```python
from build123d import *

# Parameters (mm, degrees)
SKETCH006_R     = 2.5
PAD002_DEPTH    = 9
SKETCH007_R     = 5.5
POCKET001_DEPTH = 1.85
SKETCH008_R     = 5.25
POCKET002_DEPTH = 67.1275389628
CHAMFER001_SIZE = 2.3


with BuildPart() as part:
    # Sketch006 → Pad002 (new body, symmetric)
    with BuildSketch(Plane.XY):
        with BuildLine():
            Line((20, -1.5), (20, 1.5))
            Line((20, 1.5), (7.1239047452, 1.5))
            ThreePointArc((3.9577107596, 3.0555728668), (5.3600599952, 1.9098946593), (7.1239047452, 1.5))
            ThreePointArc((3.9577107595, 3.0555728668), (-5, -2.4792e-06), (3.9577137897, -3.055568942))
            ThreePointArc((7.1239047446, -1.5), (5.3600622201, -1.9098935662), (3.9577137897, -3.055568942))
            Line((7.1239047446, -1.5), (20, -1.5))
        make_face()
        Circle(SKETCH006_R, mode=Mode.SUBTRACT)
    extrude(amount=PAD002_DEPTH, both=True)

    # Sketch007 → Pocket001 (cut, symmetric)
    with BuildSketch(Plane.XY):
        Circle(SKETCH007_R)
    extrude(amount=POCKET001_DEPTH, both=True, mode=Mode.SUBTRACT)

    # Sketch008 → Pocket002 (cut, through all)
    with BuildSketch(Plane.XY.offset(6.65)):
        Circle(SKETCH008_R)
    pocket002 = extrude(amount=POCKET002_DEPTH, mode=Mode.SUBTRACT)

    # Mirrored001: Pocket002 across XY
    add(pocket002.mirror(Plane.XY), mode=Mode.SUBTRACT)

    # Chamfer001
    chamfer001_edges = [part.edges().sort_by_distance(p)[0] for p in [
        (-2.5, 0, -6.65),
        (-2.5, 0, -1.85),
        (-2.5, 0, 6.65),
        (-2.5, 0, 1.85),
    ]]
    chamfer(chamfer001_edges, length=CHAMFER001_SIZE)


solid = part.part
```
Design review of the part built by this model. Coordinates are the model's own, in mm. A direction names the side the tool comes from. Give positions to 0.01 mm unless a question says otherwise; leave off trailing zeros. Write each loop counter-clockwise with the first axis right and the second up, starting at its lowest first coordinate (ties: lowest second). Pieces come first, ordered by that corner, then holes. Notation, with made-up numbers: (54.25, 42.5) - (64.25, 42.5) arc R24 ccw to (64.25, 52.5) - close; hole circle Ø4 at (83.5, 42.5). An arc over 180 degrees is marked (long way). Return JSON: item names as keys, results as strings. Group by question number.
(1) Machinability: for faces 5 (the flat face through (4.7, 1.9, 6.65)), 6 (the cylindrical face through (5.5, 0, 0)), 7 (the flat face through (4.7, 1.9, -6.65)), which of the approach directions +Z, -Z, +X, -X, +Y, -Y give a long, thin tool a straight path to every point of the face, cutting with its end or side? Answer none if there is none.
(2) To check wall thickness, follow probe 1 along X at (y, z) = (0, -4.2); probe 2 along X at (y, z) = (0, 2.5); probe 3 along Y at (x, z) = (13.25, -7.5). State the ranges of each line that lie inside material, in increasing order.
(3) Mouldability with a two-part tool opening along Y and no side actions: class faces 1 (the conical face through (-0.57, 2.58, -4.01)), 2 (the flat face through (5, 0, 1.85)), 3 (the flat face through (14, 1.5, 0)), 4 (the flat face through (13, -1.5, 0)) as +Y half, -Y half, draft (parallel to the pull), parting line (faces both ways), or undercut.
(4) We need section C-C, the plane x = 0. Give the boundary of the cut face in (y, z).
(5) Insertion check: pin 1 (3 mm diameter, centred on x = 7.5, z = 4.5, fed in from +Y); pin 2 (6.5 mm diameter, centred on x = 12, z = 2.5, fed in from +Y); pin 3 (3 mm diameter, centred on y = -2.5, z = -5.5, fed in from -X). Each pin has a flat end and moves straight along its axis. Give the tip position at first contact, or say it passes through.
(6) We need section B-B, the plane z = -3.5. Give the boundary of the cut face in (x, y), then the cut area to 3 significant figures.
(7) We need section A-A, the plane y = 0. Give the boundary of the cut face in (x, z), then the cut area to 3 significant figures.
(8) We need section D-D, the plane z = 0.25. Give the boundary of the cut face in (x, y).
Reported:
{
 "1": {"face 5": "+Z, -X", "face 6": "-X", "face 7": "-Z, -X"},
 "2": {"probe 1": "x = -5 to -2.5, 2.5 to 20", "probe 2": "x = -5 to -4.15, 4.15 to 20", "probe 3": "y = -1.5 to 1.5"},
 "3": {"face 1": "undercut", "face 2": "undercut", "face 3": "+Y half", "face 4": "-Y half"},
 "4": {"outline": "(-5, -6.65) - (-4.8, -6.65) - (-2.5, -4.35) - (-2.5, -4.15) - (-4.8, -1.85) - (-5, -1.85) - close; (-5, 1.85) - (-4.8, 1.85) - (-2.5, 4.15) - (-2.5, 4.35) - (-4.8, 6.65) - (-5, 6.65) - close; (2.5, -4.35) - (4.8, -6.65) - (5, -6.65) - (5, -1.85) - (4.8, -1.85) - (2.5, -4.15) - close; (2.5, 4.15) - (4.8, 1.85) - (5, 1.85) - (5, 6.65) - (4.8, 6.65) - (2.5, 4.35) - close"},
 "5": {"pin 1": "stops at y = 1.66", "pin 2": "stops at y = 1.5", "pin 3": "stops at x = -4.9"},
 "6": {"outline": "(3.96, -3.06) arc R4 cw to (7.12, -1.5) - (20, -1.5) - (20, 1.5) - (7.12, 1.5) arc R4 cw to (3.96, 3.06) arc R5 ccw (long way) to start; hole circle Ø6.3 at (0, 0)", "area": "94.1 mm2"},
 "7": {"outline": "(-5, -6.65) - (-4.8, -6.65) - (-2.5, -4.35) - (-2.5, -4.15) - (-4.8, -1.85) - (-5, -1.85) - close; (-5, 1.85) - (-4.8, 1.85) - (-2.5, 4.15) - (-2.5, 4.35) - (-4.8, 6.65) - (-5, 6.65) - close; (2.5, -4.35) - (4.8, -6.65) - (5.25, -6.65) - (5.25, -9) - (20, -9) - (20, 9) - (5.25, 9) - (5.25, 6.65) - (4.8, 6.65) - (2.5, 4.35) - (2.5, 4.15) - (4.8, 1.85) - (5.5, 1.85) - (5.5, -1.85) - (4.8, -1.85) - (2.5, -4.15) - close", "area": "294 mm2"},
 "8": {"outline": "(5.1, -2.05) arc R4 cw to (7.12, -1.5) - (20, -1.5) - (20, 1.5) - (7.12, 1.5) arc R4 cw to (5.1, 2.05) arc R5.5 cw to start"}
}
